Geometry check sheet. Reference: the model listing, model coordinates, mm. A direction names the side the tool comes from. Coordinates: 2 decimals unless noted, no trailing zeros. Write each loop counter-clockwise with the first axis right and the second up, starting at its lowest first coordinate (ties: lowest second). Pieces come first, ordered by that corner, then holes.
from build123d import *

# Parameters (mm, degrees)
BOSS_EXTRUDE2_DEPTH      = 8
BOSS_EXTRUDE2_DEPTH_BACK = 1
SKETCH1_R                = 2.5
CUT_EXTRUDE1_START       = -18
SKETCH2_R                = 2.5
CUT_EXTRUDE1_DEPTH       = 18
SKETCH3_R                = 2.75
BOSS_EXTRUDE3_DEPTH      = 13.75
SKETCH4_W                = 4.5
SKETCH4_H                = 6.5
BOSS_EXTRUDE4_DEPTH      = 15
BOSS_EXTRUDE5_DEPTH      = 8.5
SKETCH8_W                = 9
SKETCH8_H                = 6.5
BOSS_EXTRUDE6_DEPTH      = 6
SKETCH9_W                = 15.5
SKETCH9_H                = 6.5
BOSS_EXTRUDE7_DEPTH      = 21
BOSS_EXTRUDE8_DEPTH      = 8.5
CUT_EXTRUDE2_START       = -8.5
SKETCH12_R               = 3.5
CUT_EXTRUDE2_DEPTH       = 8.5
FILLET1_R                = 10
BOSS_EXTRUDE9_DEPTH      = 11
BOSS_EXTRUDE9_DEPTH_BACK = 10
SKETCH13_W               = 27.5
SKETCH13_H               = 9


with BuildPart() as part:
    # Sketch1 → Boss-Extrude2 (new, two sides: drawn at the far end of the back side and taken through both)
    with BuildSketch(Plane(origin=(0, 0, 0), x_dir=(1, 0, 0), z_dir=(0, 1, 0)).offset(-BOSS_EXTRUDE2_DEPTH_BACK)):
        with BuildLine():
            Line((5, 0), (50, 0))
            ThreePointArc((50, 0), (53.535533906, 1.464466094), (55, 5))
            Line((55, 5), (55, 50))
            ThreePointArc((55, 50), (53.535533906, 53.535533906), (50, 55))
            Line((50, 55), (5, 55))
            ThreePointArc((5, 55), (1.464466094, 53.535533906), (0, 50))
            Line((0, 50), (0, 5))
            ThreePointArc((0, 5), (1.464466094, 1.464466094), (5, 0))
        make_face()
        with Locations(Location((7.5, 47.5, 0), (0, 0, 270))):
            Circle(SKETCH1_R, mode=Mode.SUBTRACT)
        with Locations(Location((47.5, 47.5, 0), (0, 0, 270))):
            Circle(SKETCH1_R, mode=Mode.SUBTRACT)
        with Locations(Location((47.5, 7.5, 0), (0, 0, 270))):
            Circle(SKETCH1_R, mode=Mode.SUBTRACT)
        with Locations(Location((7.5, 7.5, 0), (0, 0, 270))):
            Circle(SKETCH1_R, mode=Mode.SUBTRACT)
    extrude(amount=BOSS_EXTRUDE2_DEPTH + BOSS_EXTRUDE2_DEPTH_BACK)

    # Sketch2 → Cut-Extrude1 (cut)
    with BuildSketch(Plane(origin=(0, 8, 0), x_dir=(1, 0, 0), z_dir=(0, 1, 0)).offset(CUT_EXTRUDE1_START)):
        with BuildLine():
            Line((0, 50), (0, 27.5))
            Line((0, 27.5), (55, 27.5))
            Line((55, 27.5), (55, 50))
            ThreePointArc((55, 50), (53.535533906, 53.535533906), (50, 55))
            Line((50, 55), (5, 55))
            ThreePointArc((5, 55), (1.464466094, 53.535533906), (0, 50))
        make_face()
        with Locations((7.5, 47.5)):
            Circle(SKETCH2_R, mode=Mode.SUBTRACT)
        with Locations((47.5, 47.5)):
            Circle(SKETCH2_R, mode=Mode.SUBTRACT)
    extrude(amount=CUT_EXTRUDE1_DEPTH, mode=Mode.SUBTRACT)

    # Sketch3 → Boss-Extrude3 (add)
    with BuildSketch(Plane(origin=(0, 0, -27.5), x_dir=(-1, 0, 0), z_dir=(0, 0, -1))):
        with Locations((-37.5, 3.5)):
            Circle(SKETCH3_R)
        with Locations((-17.5, 3.5)):
            Circle(SKETCH3_R)
    extrude(amount=BOSS_EXTRUDE3_DEPTH)

    # Sketch4 → Boss-Extrude4 (add)
    with BuildSketch(Plane(origin=(0, 8, 0), x_dir=(1, 0, 0), z_dir=(0, 1, 0))):
        with Locations((25.25, 20.75)):
            Rectangle(SKETCH4_W, SKETCH4_H)
        with Locations((29.75, 20.75)):
            Rectangle(SKETCH4_W, SKETCH4_H)
    extrude(amount=BOSS_EXTRUDE4_DEPTH)

    # Sketch5 → Boss-Extrude5 (add)
    with BuildSketch(Plane(origin=(0, 0, -24), x_dir=(-1, 0, 0), z_dir=(0, 0, -1))):
        with BuildLine():
            ThreePointArc((-25.636419782, 13.037388184), (-24.436298745, 14.307742745), (-24, 16))
            ThreePointArc((-24, 16), (-29.974873734, 18.474873734), (-27.5, 12.5))
            ThreePointArc((-27.5, 12.5), (-26.685966178, 12.595980474), (-25.916578842, 12.878657751))
            ThreePointArc((-25.916578842, 12.878657751), (-25.85405917, 13.094916041), (-25.636419782, 13.037388184))
        make_face()
    extrude(amount=BOSS_EXTRUDE5_DEPTH)

    # Sketch8 → Boss-Extrude6 (add)
    with BuildSketch(Plane(origin=(0, 23, 0), x_dir=(1, 0, 0), z_dir=(0, 1, 0))):
        with Locations((27.5, 20.75)):
            Rectangle(SKETCH8_W, SKETCH8_H)
    extrude(amount=BOSS_EXTRUDE6_DEPTH)

    # Sketch9 → Boss-Extrude7 (add)
    with BuildSketch(Plane(origin=(0, 8, 0), x_dir=(1, 0, 0), z_dir=(0, 1, 0))):
        with Locations((15.25, 20.75)):
            Rectangle(SKETCH9_W, SKETCH9_H)
        with Locations((39.75, 20.75)):
            Rectangle(SKETCH9_W, SKETCH9_H)
    extrude(amount=BOSS_EXTRUDE7_DEPTH)

    # Sketch10 → Boss-Extrude8 (add)
    with BuildSketch(Plane(origin=(0, 0, -24), x_dir=(-1, 0, 0), z_dir=(0, 0, -1))):
        with BuildLine():
            Line((-21, 17), (-17.5, 17))
            Line((-17.5, 17), (-14, 17))
            ThreePointArc((-14, 17), (-17.5, 20.5), (-21, 17))
        make_face()
        with BuildLine():
            Line((-17.5, 13.5), (-17.5, 17))
            Line((-17.5, 17), (-21, 17))
            ThreePointArc((-21, 17), (-19.974873734, 14.525126266), (-17.5, 13.5))
        make_face()
        with BuildLine():
            Line((-14, 17), (-17.5, 17))
            Line((-17.5, 17), (-17.5, 13.5))
            ThreePointArc((-17.5, 13.5), (-15.025126266, 14.525126266), (-14, 17))
        make_face()
        with BuildLine():
            Line((-37.5, 17), (-34, 17))
            ThreePointArc((-34, 17), (-37.5, 20.5), (-41, 17))
            Line((-41, 17), (-37.5, 17))
        make_face()
        with BuildLine():
            ThreePointArc((-37.5, 13.5), (-35.025126266, 14.525126266), (-34, 17))
            Line((-34, 17), (-37.5, 17))
            Line((-37.5, 17), (-37.5, 13.5))
        make_face()
        with BuildLine():
            Line((-37.5, 13.5), (-37.5, 17))
            Line((-37.5, 17), (-41, 17))
            ThreePointArc((-41, 17), (-39.974873734, 14.525126266), (-37.5, 13.5))
        make_face()
    extrude(amount=BOSS_EXTRUDE8_DEPTH)

    # Sketch12 → Cut-Extrude2 (cut)
    with BuildSketch(Plane(origin=(0, 0, -32.5), x_dir=(-1, 0, 0), z_dir=(0, 0, -1)).offset(CUT_EXTRUDE2_START)):
        with Locations((-27.5, 16)):
            Circle(SKETCH12_R)
    extrude(amount=CUT_EXTRUDE2_DEPTH, mode=Mode.SUBTRACT)

    # Fillet1
    fillet1_edges = [part.edges().sort_by_distance(p)[0] for p in [
        (7.5, 29, -20.75),
        (47.5, 29, -20.75),
    ]]
    fillet(fillet1_edges, radius=FILLET1_R)

    # Sketch13 → Boss-Extrude9 (add, two sides: drawn at the far end of the back side and taken through both)
    with BuildSketch(Plane.ZY.offset(-BOSS_EXTRUDE9_DEPTH_BACK)):
        with Locations((-13.75, 3.5)):
            Rectangle(SKETCH13_W, SKETCH13_H)
    extrude(amount=BOSS_EXTRUDE9_DEPTH + BOSS_EXTRUDE9_DEPTH_BACK)


solid = part.part
1. Sectioned sample at C-C, the plane z = -6. Record the boundary of the cut face in (x, y), and give its area (3 significant figures).
Computed values:
outline: (-11, -1) - (45.5, -1) - (45.5, 8) - (-11, 8) - close; (49.5, -1) - (55, -1) - (55, 8) - (49.5, 8) - close
area: 558 mm2
2. Sectioned sample at A-A, the plane z = -31. Record the boundary of the cut face in (x, y).
Computed values:
outline: circle Ø7 at (17.5, 17); circle Ø5.5 at (17.5, 3.5); circle Ø7 at (37.5, 17); circle Ø5.5 at (37.5, 3.5)
3. Sectioned sample at D-D, the plane x = 32. Record the boundary of the cut face in (y, z), and give its area (3 significant figures).
Computed values:
outline: (-1, -27.5) - (8, -27.5) - (8, -24) - (29, -24) - (29, -17.5) - (8, -17.5) - (8, 0) - (-1, 0) - close
area: 384 mm2
4. Draft check along X on faces 6 (the flat face through (55, 3, -16)), 7 (the flat face through (-11, 4, -14)), 8 (the cylindrical face through (40.247, 3.621, -34.279)). Enter one of: released by +X, released by -X, zero draft, split by the parting line, or undercut.
Computed values:
face 6: released by +X
face 7: released by -X
face 8: undercut
5. Gauge pin test, flat ends, axial feed: pin 1 Ø5.5 at (x, y) = (17, 17) entering from -Z; pin 2 Ø4 at (y, z) = (22.5, -21) entering from +X; pin 3 Ø10 at (x, z) = (17, -30) entering from +Y. Record the tip position at first contact, or that the pin passes through.
Computed values:
pin 1: stops at z = -32.5
pin 2: stops at x = 47.39
pin 3: stops at y = 20.5
6. Thickness scan on line 1 along X through (y, z) = (2.25, -7.5); line 2 along Y through (x, z) = (44.5, -8); line 3 along Z through (x, y) = (10.5, 23.5). Record the ranges inside material, lowest first.
Computed values:
line 1: x = -11 to 45, 50 to 55
line 2: y = -1 to 8
line 3: z = -24 to -17.5
7. Sectioned sample at B-B, the plane y = 3.5. Record the boundary of the cut face in (x, z).
Computed values:
outline: (-11, -27.5) - (14.75, -27.5) - (14.75, -41.25) - (20.25, -41.25) - (20.25, -27.5) - (34.75, -27.5) - (34.75, -41.25) - (40.25, -41.25) - (40.25, -27.5) - (55, -27.5) - (55, -5) arc R5 ccw to (50, 0) - (-11, 0) - close; hole circle Ø5 at (47.5, -7.5)
8. Access from +Z, -Z, +X, -X, +Y, -Y to the whole of each face (thin tool, end or side, straight path). Record for faces 1 (the flat face through (7.5, 13, -21)), 2 (the cylindrical face through (19.682, 1.827, -34.279)), 3 (the flat face through (27, 18, -17.5)), 4 (the flat face through (47.5, 13, -21)), 5 (the flat face through (38, 17, -32.5)).
Computed values:
face 1: +Z, -Z, -X, +Y
face 2: -Z
face 3: +Z, +X, -X, +Y
face 4: +Z, -Z, +X, +Y
face 5: -Z, +X, -X, +Y
